For this review, take the finished solid that the model builds, in its own axes (mm). Face numbers are marked on the shaded views. A direction names the side the tool comes from. Give positions to 0.01 mm unless a question says otherwise; leave off trailing zeros. Write each loop counter-clockwise with the first axis right and the second up, starting at its lowest first coordinate (ties: lowest second). Pieces come first, ordered by that corner, then holes.
1) We need section A-A on z = 11. Give the boundary of the cut face in (x, y), and give its area (3 significant figures).
2) Wall thickness on line 1 along Z through (x, y) = (11.5, -23); line 2 along Z through (x, y) = (15.5, -12); line 3 along X through (y, z) = (-7.5, 21): over which ranges is each line inside the solid? List them lowest first.
3) Machinability: for the marked faces 1, 2, 3 and 4, which of the approach directions +Z, -Z, +X, -X, +Y, -Y give a long, thin tool a straight path to every point of the face, cutting with its end or side? Answer none if there is none.
4) For P1, Ø1, axis at y = -6.5, z = 25, coming from the +X side; P2, Ø5, axis at y = -2.5, z = 13, coming from the -X side; P3, Ø1, axis at x = 1.5, z = 28.5, coming from the -Y side, all flat-tipped, find the tip position at first contact; note any pin that passes through.
5) We need section B-B on z = 24. Give the boundary of the cut face in (x, y), and give its area (3 significant figures).
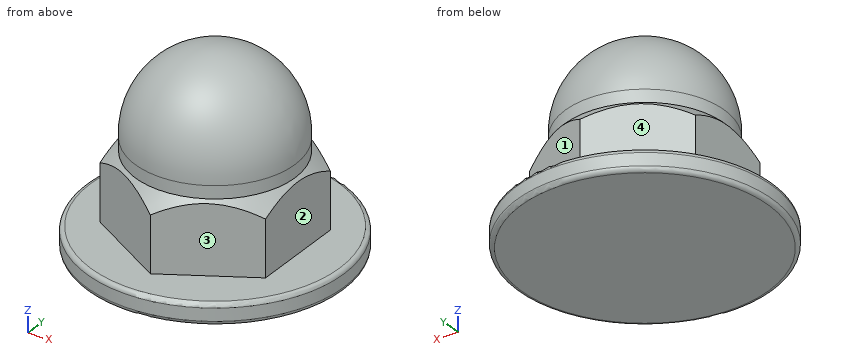
from build123d import *

# Parameters (mm, degrees)
SKETCH1_R           = 30.453013084
BOSS_EXTRUDE1_DEPTH = 5
BOSS_EXTRUDE2_DEPTH = 17
SKETCH3_R           = 36.437835874
SKETCH3_R_2         = 18.912930376
CUT_EXTRUDE1_DEPTH  = 17
CUT_EXTRUDE1_TAPER  = 45
SKETCH4_R           = 18.912930376
BOSS_EXTRUDE3_DEPTH = 3
DOME1_FACE_RADIUS   = 18.912930376
DOME1_HEIGHT        = 20
FILLET1_R           = 1
FILLET2_R           = 1


with BuildPart() as part:
    # Sketch1 → Boss-Extrude1 (new body)
    with BuildSketch(Plane.XY):
        Circle(SKETCH1_R)
    extrude(amount=BOSS_EXTRUDE1_DEPTH)

    # Sketch2 → Boss-Extrude2 (add)
    with BuildSketch(Plane.XY.offset(5)):
        Polygon((0, 22.618579174), (-19.588264162, 11.309289587), (-19.588264162, -11.309289587), (0, -22.618579174), (19.588264162, -11.309289587), (19.588264162, 11.309289587), align=None)
    extrude(amount=BOSS_EXTRUDE2_DEPTH)

    # Sketch3 → Cut-Extrude1 (cut)
    with BuildSketch(Plane.XY.offset(22)):
        Circle(SKETCH3_R)
        Circle(SKETCH3_R_2, mode=Mode.SUBTRACT)
    extrude(amount=-CUT_EXTRUDE1_DEPTH, taper=CUT_EXTRUDE1_TAPER, mode=Mode.SUBTRACT)

    # Sketch4 → Boss-Extrude3 (add)
    with BuildSketch(Plane.XY.offset(22)):
        Circle(SKETCH4_R)
    extrude(amount=BOSS_EXTRUDE3_DEPTH)

    # Dome1: a dome of height H over a round flat face of radius A is a cap of a sphere of radius (A * A + H * H) / (2 * H)
    dome1_r = (DOME1_FACE_RADIUS * DOME1_FACE_RADIUS + DOME1_HEIGHT * DOME1_HEIGHT) / (2 * DOME1_HEIGHT)
    dome1_base = Plane((0, 0, 25), z_dir=(0, 0, 1))
    with Locations(dome1_base.offset(DOME1_HEIGHT - dome1_r)):
        dome1_ball = Sphere(dome1_r, mode=Mode.PRIVATE)
    add(split(dome1_ball, bisect_by=dome1_base, keep=Keep.TOP, mode=Mode.PRIVATE))

    # Fillet1
    fillet1_edges = [part.edges().sort_by_distance(p)[0] for p in [
        (-30.453013084, 0, 5),
    ]]
    fillet(fillet1_edges, radius=FILLET1_R)

    # Fillet2
    fillet2_edges = [part.edges().sort_by_distance(p)[0] for p in [
        (-30.453013084, 0, 0),
    ]]
    fillet(fillet2_edges, radius=FILLET2_R)


solid = part.part
Results list:
1. outline: (-19.59, -11.31) - (0, -22.62) - (19.59, -11.31) - (19.59, 11.31) - (0, 22.62) - (-19.59, 11.31) - close
1. area: 1,330 mm2
2. line 1: z = 0 to 5
2. line 2: z = 0 to 21.31
2. line 3: x = -18.45 to 18.45
3. face 1: +Z, +X, +Y
3. face 2: +Z, +X, +Y, -Y
3. face 3: +Z, +X, -Y
3. face 4: +Z, -X, +Y
4. P1: stops at x = 17.94
4. P2: stops at x = -19.59
4. P3: stops at y = -18.79
5. outline: circle Ø37.83 at (0, 0)
5. area: 1,120 mm2
